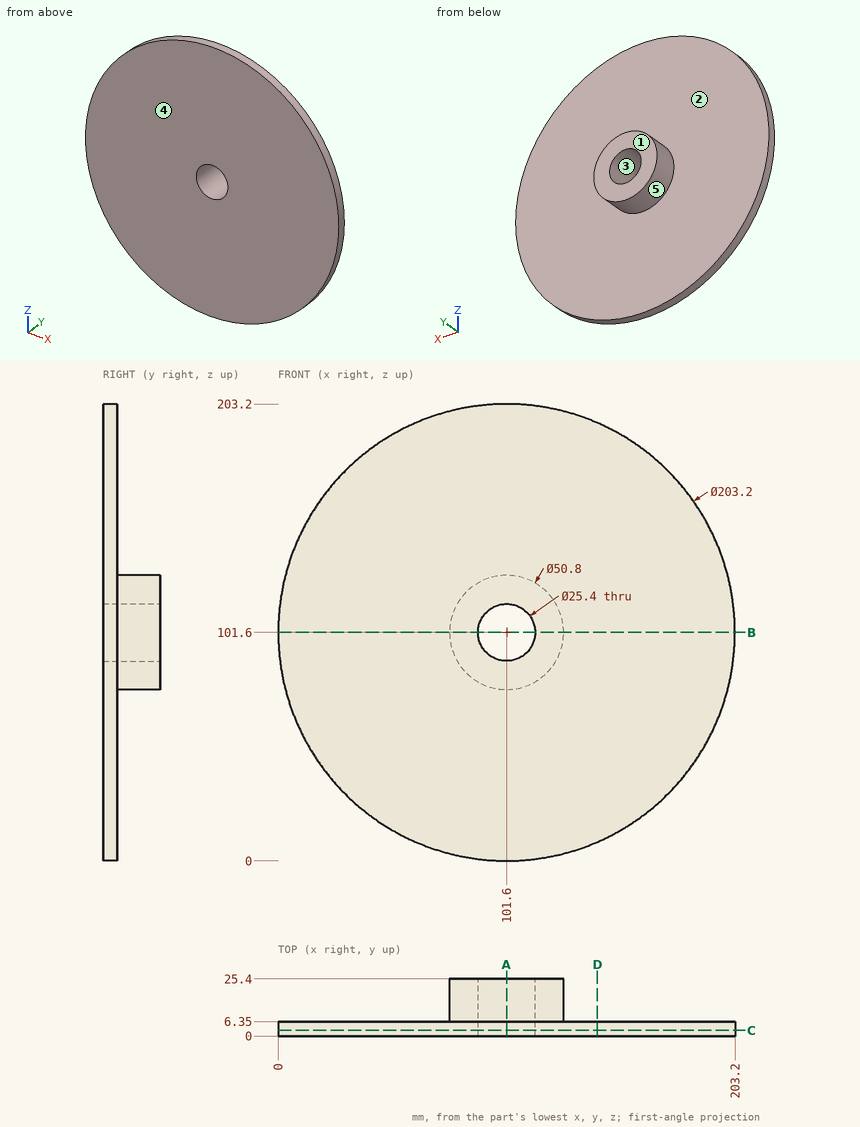
Can you work these out from the drawing? Everything is in mm from the part's minimum corner. A direction names the side the tool comes from. Round coordinates to 2 decimals unless told otherwise and drop trailing zeros. Order: outer loops, then holes, each group sorted by start corner. A loop starts at its lowest first (then second) coordinate and runs counter-clockwise, first axis right, second up. Notation, with made-up numbers: (8, 80.25) -> (27, 80.25) arc R23 cw to (27, 110.25) -> close; hole circle Ø3 at (-15.5, -30). An arc over 180 degrees is marked (long way). Use CSV: the item, a comma, the result in double quotes.
1. I want a section at C-C on y = 2.5. List the corners of the cut face in (x, z) for me, and give its area (3 significant figures).
Recorded:
outline,"circle Ø203.2 at (101.6, 101.6); hole circle Ø25.4 at (101.6, 101.6)"
area,"31,900 mm2"
2. I'm going to push flat-ended pins straight in: P1, Ø12, axis at x = 140.5, y = 17.5, coming from the +Z side; P2, Ø10, axis at y = 7, z = 63, coming from the +X side; P3, Ø8, axis at x = 45.5, z = 150, coming from the +Y side; P4, Ø3, axis at y = 4, z = 90.5, coming from the +X side. Where does each tip first touch, or does it pass through?
Recorded:
P1,"passes through"
P2,"stops at x = 197.47"
P3,"stops at y = 6.35"
P4,"stops at x = 202.75"
3. I want a section at B-B on z = 101.6. List the corners of the cut face in (x, y) for me, and give its area (3 significant figures).
Recorded:
outline,"(0, 0) -> (88.9, 0) -> (88.9, 25.4) -> (76.2, 25.4) -> (76.2, 6.35) -> (0, 6.35) -> close; (114.3, 0) -> (203.2, 0) -> (203.2, 6.35) -> (127, 6.35) -> (127, 25.4) -> (114.3, 25.4) -> close"
area,"1,610 mm2"
4. I want a section at D-D on x = 142. List the corners of the cut face in (y, z) for me, and give its area (3 significant figures).
Recorded:
outline,"(0, 8.38) -> (6.35, 8.38) -> (6.35, 194.82) -> (0, 194.82) -> close"
area,"1,180 mm2"
5. Which directions (+Z, -Z, +X, -X, +Y, -Y) give clear straight access to the entire face, cutting with the end or side of a thin tool? Please do the marked faces 1 and 2.
Recorded:
face 1,"+Z, -Z, +X, -X, +Y"
face 2,"+Y"
6. I need wall thicknesses on line 1 along Z through (x, y) = (101.6, 8.25); line 2 along Y through (x, z) = (33, 119.5); line 3 along Z through (x, y) = (103.5, 17.75). Which ranges of each line are inside material? Lowest first, please.
Recorded:
line 1,"z = 76.2 to 88.9, 114.3 to 127"
line 2,"y = 0 to 6.35"
line 3,"z = 76.27 to 89.04, 114.16 to 126.93"
7. Thinking about a two-plate mould opening in X: for the marked faces 3, 4 and 5, which applies, pulls with the +X half, pulls with the -X half, needs draft (parallel to the pull), parting line crosses it, or undercut?
Recorded:
face 3,"undercut"
face 4,"needs draft"
face 5,"parting line crosses it"
8. I want a section at A-A on x = 101.6. List the corners of the cut face in (y, z) for me.
Recorded:
outline,"(0, 0) -> (6.35, 0) -> (6.35, 76.2) -> (25.4, 76.2) -> (25.4, 88.9) -> (0, 88.9) -> close; (0, 114.3) -> (25.4, 114.3) -> (25.4, 127) -> (6.35, 127) -> (6.35, 203.2) -> (0, 203.2) -> close"
